Can you work these out from the model? Positions are in its coordinate system, mm. Face numbers are marked on the shaded views. A direction names the side the tool comes from. Give positions to 0.01 mm unless a question says otherwise; leave off trailing zeros. Order: outer loops, then holes, each group sorted by start corner. A loop starts at its lowest first (then second) coordinate and runs counter-clockwise, first axis right, second up. Notation, with made-up numbers: M 73,26.5 L 105,26.5 A20 ccw 105,38.5 Z; hole C -34.5,10.5 d11. An arc over 180 degrees is marked long. Use a Markdown table: item, result. Add a question column.
from build123d import *

# Parameters (mm, degrees)
EXTRUDE_THIN1_DEPTH = 400
SKETCH2_R           = 3
CUT_EXTRUDE1_DEPTH  = 10
LPATTERN1_COUNT     = 2
LPATTERN1_PITCH     = 370
SKETCH3_R           = 3
CUT_EXTRUDE2_DEPTH  = 10
LPATTERN2_COUNT     = 2
LPATTERN2_PITCH     = 370


with BuildPart() as part:
    # Sketch1 → Extrude-Thin1 (new body)
    with BuildSketch(Plane.XY):
        Polygon((0, 0), (-27, 0), (-27, -27), (-30, -27), (-30, 3), (0, 3), align=None)
    extrude(amount=EXTRUDE_THIN1_DEPTH)

    # Sketch2 → Cut-Extrude1 (cut)
    with BuildSketch(Plane(origin=(0, 3, 0), x_dir=(1, 0, 0), z_dir=(0, 1, 0))):
        with Locations(Location((-15, -15, 0), (0, 0, 270))):
            Circle(SKETCH2_R)
    cut_extrude1 = extrude(amount=-CUT_EXTRUDE1_DEPTH, mode=Mode.SUBTRACT)

    # LPattern1: Cut-Extrude1 ×2
    with Locations(*[(0, 0, i * LPATTERN1_PITCH) for i in range(1, LPATTERN1_COUNT)]):
        add(cut_extrude1, mode=Mode.SUBTRACT)

    # Sketch3 → Cut-Extrude2 (cut)
    with BuildSketch(Plane.ZY.offset(30)):
        with Locations((15, -12)):
            Circle(SKETCH3_R)
    cut_extrude2 = extrude(amount=-CUT_EXTRUDE2_DEPTH, mode=Mode.SUBTRACT)

    # LPattern2: Cut-Extrude2 ×2
    with Locations(*[(0, 0, i * LPATTERN2_PITCH) for i in range(1, LPATTERN2_COUNT)]):
        add(cut_extrude2, mode=Mode.SUBTRACT)


solid = part.part
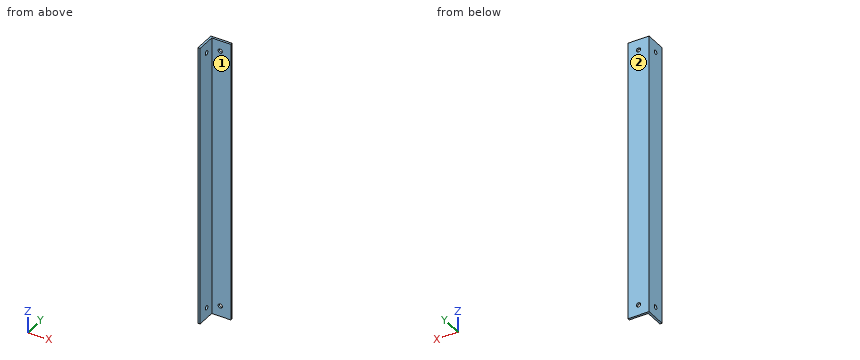
1. On a 3-axis mill with a long thin cutter (end or side, diameter ignored), from which of +Z, -Z, +X, -X, +Y, -Y can I reach the whole of each face in a straight line? I mean the marked faces 1 and 2. Say none if no direction works.
2. I need wall thicknesses on L1, parallel to X at y = 1.3, z = 385; L2, parallel to Y at x = -10.25, z = 16; L3, parallel to X at y = -22.75, z = 299. Which ranges of each line are inside material? Lowest first, please. Write a range as [from, to].
3. If we section it at B-B, the plane x = -8.25: List the corners of the cut face in (y, z) for me.
4. Will these pins go through, and if not, where does the flat tip stop? pin 1 (6 mm diameter, centred on x = -7, y = -2, fed in from +Z); pin 2 (4 mm diameter, centred on x = -22.5, z = 164, fed in from -Y); pin 3 (3 mm diameter, centred on y = -12.5, z = 82.5, fed in from +X).
5. If we section it at A-A, the plane z = 26: List the corners of the cut face in (x, y) for me, then the cut area to 3 significant figures.
Geometry results:
| question | item | result |
|---|---|---|
| 1 | face 1 | +Z, -Z, +X, -Y |
| 1 | face 2 | +Z, -Z, +X, -X, +Y |
| 2 | L1 | x = [-30, -18], [-12, 0] |
| 2 | L2 | y = [0, 3] |
| 2 | L3 | x = [-30, -27] |
| 3 | outline | M 0,0 L 3,0 L 3,400 L 0,400 Z |
| 4 | pin 1 | stops at z = 400 |
| 4 | pin 2 | stops at y = 0 |
| 4 | pin 3 | stops at x = -27 |
| 5 | outline | M -30,-27 L -27,-27 L -27,0 L 0,0 L 0,3 L -30,3 Z |
| 5 | area | 171 mm^2 |
